Autodesk Inventor part; units mm, degrees
ref_plane "YZ Plane" through (0, 0, 0) normal (1, 0, 0) x (0, 1, 0)
ref_plane "XZ Plane" through (0, 0, 0) normal (0, 1, 0) x (-1, 0, 0)
ref_plane "XY Plane" through (0, 0, 0) normal (0, 0, 1) x (1, 0, 0)
sketch "スケッチ1" plane through (0, 0, 0) normal (1, 0, 0) x (0, 1, 0)
  circle A0 centre (0, 0) radius 12.5
  dimension "d0" = 25
extrude "押し出し1" add sketch "スケッチ1" along normal blind 28.5
sketch "スケッチ2" plane through (28.5, 0, 0) normal (1, 0, 0) x (0, 0, -1)
  point P0 (0, 0)
  point P1 (0, 0)
hole "穴1" at (28.5, 0, 0) direction (-1, 0, 0) diameter 6 end through all
sketch "スケッチ3" plane through (0, 0, 0) normal (-1, 0, 0) x (0, 0, 1)
  circle A0 centre (0, 0) radius 3
hole "穴2" at (0, 0, 0) direction (1, 0, 0) diameter 8 depth 17
properties part number "OC25S-6-8" material "アルミニウム 6061"
Geometry: final body of the model. Coordinates: model frame, mm. A direction names the side the tool comes from. Round coordinates to 2 decimals unless told otherwise and drop trailing zeros. Loops run counter-clockwise (first coordinate to the right, second up) from the corner with the lowest first, then second, coordinate; pieces in that order, holes last. Notation, with made-up numbers: M -22.5,-29.75 L 10.5,-29.75 A23 ccw 10.5,1.25 Z; hole C 46.5,12.5 d9. An arc over 180 degrees is marked long. Put each result on its own line as item: value. Start each with the question number.
(1) Draft query along Z for faces 3 (the face through (17, -3, 1)), 4 (the face through (14.05, 11.923, -3.755)), 5 (the face through (0, -3, 3)), 6 (the face through (23, 0, 3)). Return one class per face: +Z half, -Z half, draft (parallel to the pull), parting line (faces both ways), or undercut.
(2) Section query C-C (x = 8). Return loops of the section in (y, z), then the cut area to 3 significant figures.
(3) Set-up query: faces 1 (the face through (8.619, 3.905, -0.867)), 2 (the face through (28.5, 3, -3)). Return all of +Z, -Z, +X, -X, +Y, -Y with unobstructed straight access to the full face (end or side cutting, diameter ignored); none if empty.
(4) Section query D-D (z = -7.5). Return loops of the section in (x, y), then the cut area to 3 significant figures.
(5) Material intervals for line 1 along Z through (x, y) = (10, 0); line 2 along Z through (x, y) = (23.75, 0); line 3 along X through (y, z) = (-1.5, -2.75), sorted ascending. Write a range as [from, to].
(6) Contact query for flat-ended pins moving along their axis: pin 1 Ø10 at (x, z) = (16, 0.5) entering from -Y; pin 2 Ø4 at (x, y) = (6, 8) entering from -Z; pin 3 Ø5.5 at (y, z) = (0, 0) entering from +X; pin 4 Ø3 at (x, y) = (24.5, -8) entering from +Z. Output: stop coordinate, or through.
(7) Section query A-A (z = 0). Return loops of the section in (x, y).
Findings below:
1. face 3: undercut
1. face 4: parting line
1. face 5: draft
1. face 6: undercut
2. outline: C 0,0 d25; hole C 0,0 d8
2. area: 441 mm2
3. face 1: -X
3. face 2: +Z, -Z, +X, +Y, -Y
4. outline: M 0,-10 L 28.5,-10 L 28.5,10 L 0,10 Z
4. area: 570 mm2
5. line 1: z = [-12.5, -4], [4, 12.5]
5. line 2: z = [-12.5, -3], [3, 12.5]
5. line 3: x = [17, 28.5]
6. pin 1: stops at y = -12.5
6. pin 2: stops at z = -10.97
6. pin 3: passes through
6. pin 4: stops at z = 10.68
7. outline: M 0,-12.5 L 28.5,-12.5 L 28.5,-3 L 17,-3 L 17,-4 L 0,-4 Z; M 0,4 L 17,4 L 17,3 L 28.5,3 L 28.5,12.5 L 0,12.5 Z
